from build123d import *

# Parameters (mm, degrees)
SKETCH1_W                                    = 25.5
SKETCH1_H                                    = 38
BOSS_EXTRUDE1_DEPTH                          = 4
CUT_EXTRUDE1_REACH                           = 42.281
SKETCH2_W                                    = 12
SKETCH2_H                                    = 1.5
CSK_FOR_M4_COUNTERSUNK_FLAT_HEAD_SCR_2_COUNT = 2
CSK_FOR_M4_COUNTERSUNK_FLAT_HEAD_SCR_2_PITCH = 20
M3_CLEARANCE_HOLE1_D                         = 3.1
HOLE1_D                                      = 4.2
FILLET1_R                                    = 1


with BuildPart() as part:
    # Sketch1 → Boss-Extrude1 (new body)
    with BuildSketch(Plane.XY):
        Rectangle(SKETCH1_W, SKETCH1_H)
    extrude(amount=BOSS_EXTRUDE1_DEPTH)

    # Sketch2 → Cut-Extrude1 (cut, up to next)
    with BuildSketch(Plane(origin=(0, 19, 0), x_dir=(1, 0, 0), z_dir=(0, 1, 0)), mode=Mode.PRIVATE) as cut_extrude1_sk1:
        with Locations((-6.75, -0.75)):
            Rectangle(SKETCH2_W, SKETCH2_H)
    cut_extrude1_tool1 = extrude(cut_extrude1_sk1.sketch, amount=-CUT_EXTRUDE1_REACH, mode=Mode.PRIVATE) & part.part
    add(cut_extrude1_tool1.solids().sort_by_distance((-6.75, 19, 0.75))[0], mode=Mode.SUBTRACT)

    # Sketch5 → CSK for M4 Countersunk Flat Head Screw1 (revolve, cut)
    with BuildSketch(Plane(origin=(4.75, 10, 0), x_dir=(0, 1, 0), z_dir=(1, 0, 0))):
        Polygon((0, 0), (0, 4), (2.275, 4), (2.25, 3.975), (2.25, 2.45), (4.7, 0), align=None)
    csk_for_m4_countersunk_flat_head_screw1 = revolve(axis=Axis((4.75, 10, -6.35), (0, 0, 1)), mode=Mode.SUBTRACT)

    # CSK for M4 Countersunk Flat Head Scr 2: CSK for M4 Countersunk Flat Head Screw1 ×2
    with Locations(*[(0, -i * CSK_FOR_M4_COUNTERSUNK_FLAT_HEAD_SCR_2_PITCH, 0) for i in range(1, CSK_FOR_M4_COUNTERSUNK_FLAT_HEAD_SCR_2_COUNT)]):
        add(csk_for_m4_countersunk_flat_head_screw1, mode=Mode.SUBTRACT)

    # M3 Clearance Hole1 (through all)
    with Locations(Plane(origin=(0, 0, 1.5), x_dir=(-1, 0, 0), z_dir=(0, 0, -1))):
        with Locations((9.75, -16.35), (9.75, 16.35)):
            Hole(M3_CLEARANCE_HOLE1_D / 2)

    # Hole1 (through all)
    with Locations(Plane(origin=(0, 0, 1.5), x_dir=(-1, 0, 0), z_dir=(0, 0, -1))):
        with Locations((9.75, -3.3), (9.75, 3.3)):
            Hole(HOLE1_D / 2)

    # Fillet1
    fillet1_edges = [part.edges().sort_by_distance(p)[0] for p in [
        (-12.75, 19, 2.75),
        (12.75, 19, 2),
        (12.75, -19, 2),
        (-12.75, -19, 2.75),
    ]]
    fillet(fillet1_edges, radius=FILLET1_R)


solid = part.part
Verification items for the finished model (mm, model axes). A direction names the side the tool comes from. Coordinates: 2 decimals unless noted, no trailing zeros. Write each loop counter-clockwise with the first axis right and the second up, starting at its lowest first coordinate (ties: lowest second). Pieces come first, ordered by that corner, then holes. Notation, with made-up numbers: M -1.5,35 L 34.5,35 A32 ccw 34.5,70 Z; hole C 69.5,-32.75 d1. An arc over 180 degrees is marked long. Use a Markdown table: item, result.
Q1. Sectioned sample at A-A, the plane y = 16.35. Record the boundary of the cut face in (x, z), plus the area to 4 significant figures.
Reply:
| item | result |
|---|---|
| outline | M -12.75,1.5 L -11.3,1.5 L -11.3,4 L -12.75,4 Z; M -8.2,1.5 L -0.75,1.5 L -0.75,0 L 12.75,0 L 12.75,4 L -8.2,4 Z |
| area | 76.25 mm² |
Q2. Set-up check for faces 1 (the face through (6.212, -11.907, 2.297)), 2 (the face through (-0.75, 0, 1)): record each of +Z, -Z, +X, -X, +Y, -Y from which the full face is reachable in a straight line by a thin tool's end or side.
Reply:
| item | result |
|---|---|
| face 1 | -Z |
| face 2 | -Z, -X, +Y, -Y |
Q3. Go/stop test with flat-tipped pins: P1, Ø4, axis at x = -9.75, y = 16.35, coming from the -Z side; P2, Ø1.2, axis at y = 1.5, z = 1, coming from the -X side; P3, Ø4, axis at x = 4.75, y = -10, coming from the -Z side; P4, Ø2, axis at x = 2, y = -9, coming from the -Z side. Record where each tip stops, or that it passes through.
Reply:
| item | result |
|---|---|
| P1 | stops at z = 1.5 |
| P2 | stops at x = -12.75 |
| P3 | passes through |
| P4 | stops at z = 0.77 |
Q4. Sectioned sample at C-C, the plane z = 1.1. Record the boundary of the cut face in (x, y), plus the area to 3 significant figures.
Reply:
| item | result |
|---|---|
| outline | M -0.75,-19 L 11.75,-19 A1 ccw 12.75,-18 L 12.75,18 A1 ccw 11.75,19 L -0.75,19 Z; hole C 4.75,-10 d7.2; hole C 4.75,10 d7.2 |
| area | 431 mm² |
Q5. Sectioned sample at D-D, the plane x = -9.75. Record the boundary of the cut face in (y, z).
Reply:
| item | result |
|---|---|
| outline | M -19,1.5 L -17.9,1.5 L -17.9,4 L -19,4 Z; M -14.8,1.5 L -5.4,1.5 L -5.4,4 L -14.8,4 Z; M -1.2,1.5 L 1.2,1.5 L 1.2,4 L -1.2,4 Z; M 5.4,1.5 L 14.8,1.5 L 14.8,4 L 5.4,4 Z; M 17.9,1.5 L 19,1.5 L 19,4 L 17.9,4 Z |
Q6. Sectioned sample at B-B, the plane x = 4.75. Record the boundary of the cut face in (y, z) (3 decimals).
Reply:
| item | result |
|---|---|
| outline | M -19,0 L -14.7,0 L -12.25,2.45 L -12.25,3.975 L -12.275,4 L -19,4 Z; M -7.75,2.45 L -5.3,0 L 5.3,0 L 7.75,2.45 L 7.75,3.975 L 7.725,4 L -7.725,4 L -7.75,3.975 Z; M 12.25,2.45 L 14.7,0 L 19,0 L 19,4 L 12.275,4 L 12.25,3.975 Z |
Q7. Draft check along Y on faces 3 (the face through (-12.465, -18.699, 2.768)), 4 (the face through (0, 0, 4)), 5 (the face through (-12.465, 18.699, 2.768)), 6 (the face through (4.03, 12.29, 2.3)). Enter one of: +Y half, -Y half, draft (parallel to the pull), parting line (faces both ways), or undercut.
Reply:
| item | result |
|---|---|
| face 3 | -Y half |
| face 4 | draft |
| face 5 | +Y half |
| face 6 | undercut |
Q8. Thickness scan on line 1 (Y direction, x = -9.75, z = 3.4); line 2 (Y direction, x = 4.75, z = 3.15); line 3 (Y direction, x = 3, z = 1.55). Record the ranges inside material, lowest first.
Reply:
| item | result |
|---|---|
| line 1 | y = -19 to -17.9, -14.8 to -5.4, -1.2 to 1.2, 5.4 to 14.8, 17.9 to 19 |
| line 2 | y = -19 to -12.25, -7.75 to 7.75, 12.25 to 19 |
| line 3 | y = -19 to -12.62, -7.38 to 7.38, 12.62 to 19 |
